```python
from build123d import *

# Parameters (mm, degrees)
F2_R     = 1.5
F3_R     = 8
F4_DEPTH = 43.001
F5_W     = 8.1
F5_H     = 2.3
F7_SIZE  = 1


with BuildPart() as f1:
    # F0 (on Front) → F1 (revolve)
    with BuildSketch(Plane.XZ):
        Polygon((-4, 0), (0, 0), (0, 43), (-6.9282032303, 43), (-6.9282032303, 36), (-4, 36), align=None)
    revolve(axis=Axis((0, 0, 24.3542883545), (0, 0, 1)))

    # F2
    f2_edges = [f1.edges().sort_by_distance(p)[0] for p in [
        (6.928203, 0, 43),
    ]]
    fillet(f2_edges, radius=F2_R)

    # F3 (on face) → F4 (cut, through all)
    with BuildSketch(Plane.XY.offset(43)):
        Circle(F3_R)
        Polygon((0, -6.9282032303), (-6, -3.4641016151), (-6, 3.4641016151), (0, 6.9282032303), (6, 3.4641016151), (6, -3.4641016151), align=None, mode=Mode.SUBTRACT)
    extrude(amount=-F4_DEPTH, mode=Mode.SUBTRACT)

    # F5 (on Front) → F6 (revolve)
    with BuildSketch(Plane.XZ):
        with Locations((-4.05, 37.15)):
            Rectangle(F5_W, F5_H)
    revolve(axis=Axis((0, 0, 29.9482884184), (0, 0, -1)))

    # F7
    f7_edges = [f1.edges().sort_by_distance(p)[0] for p in [
        (4, 0, 0),
    ]]
    chamfer(f7_edges, length=F7_SIZE)


solid = f1.part
```
Part model, mm, in its own coordinate system. A direction names the side the tool comes from. Give positions to 0.01 mm unless a question says otherwise; leave off trailing zeros. Order: outer loops, then holes, each group sorted by start corner. A loop starts at its lowest first (then second) coordinate and runs counter-clockwise, first axis right, second up. Notation, with made-up numbers: M 30,-35 L 81,-35 A9 cw 81,-26 Z; hole C 54.25,5 d6. An arc over 180 degrees is marked long. Use a Markdown table: item, result. Add a question column.
(1) 3-axis set-ups, long thin cutter, end or side, ignore diameter. For faces 1 (the face through (4, 5, 38.3)), 2 (the face through (6, 0, 41)), 3 (the face through (3.042, -5.172, 40.626)), 4 (the face through (0.867, 3.905, 18.255)), 5 (the face through (-3.042, 5.172, 40.626)): which of +Z, -Z, +X, -X, +Y, -Y reach the whole face in a straight line?
(2) Drop flat-ended pins along their axis: P1, Ø1, axis at y = -1.5, z = 24, coming from the -X side; P2, Ø1.5, axis at x = 6, z = 13, coming from the +Y side; P3, Ø1.4, axis at y = 0, z = 41.5, coming from the +X side; P4, Ø3, axis at y = 4.5, z = 5, coming from the +X side. Give the stop position or say it passes through.
(3) Saw through at A-A, the plane y = 0. Give the cut face in (x, z).
(4) Saw through at B-B, the plane z = 26. Give the cut face in (x, y).
(5) Probe line 1 along Z through (x, y) = (4.75, 6.25); line 2 along Z through (x, y) = (-0.75, -4.5); line 3 along Y through (x, z) = (-2, 13.5). List the from-to ranges inside material, lowest first. Write a range as [from, to].
Answer key:
| question | item | result |
|---|---|---|
| 1 | face 1 | +Z |
| 1 | face 2 | +Z, +X, +Y, -Y |
| 1 | face 3 | +Z, +X, -Y |
| 1 | face 4 | -Z |
| 1 | face 5 | +Z, -X, +Y |
| 2 | P1 | x = -3.87 |
| 2 | P2 | through |
| 2 | P3 | x = 6 |
| 2 | P4 | x = 2.65 |
| 3 | outline | M -8.1,36 L -4,36 L -4,1 L -3,0 L 3,0 L 4,1 L 4,36 L 8.1,36 L 8.1,38.3 L 6,38.3 L 6,42.89 A1.5 ccw 5.43,43 L -5.43,43 A1.5 ccw -6,42.89 L -6,38.3 L -8.1,38.3 Z |
| 4 | outline | C 0,0 d8 |
| 5 | line 1 | [36, 38.3] |
| 5 | line 2 | [36, 43] |
| 5 | line 3 | [-3.46, 3.46] |
